```python
from build123d import *

# Parameters (mm, degrees)
SKETCH1_W                                  = 100
SKETCH1_H                                  = 40
BOSS_EXTRUDE1_DEPTH                        = 5
SKETCH2_R                                  = 3
CUT_EXTRUDE1_DEPTH                         = 55.083269132
MIRROR1_AT_THE_SECOND_PLANE_COPY_1_SKETC_R = 3
MIRROR1_AT_THE_SECOND_PLANE_COPY_1_DEPTH   = 55.083269132
FLEX1_START                                = 1.366197724
FLEX1_OUTLINE_W                            = 5
FLEX1_OUTLINE_H                            = 40
FLEX1_DEPTH                                = 48.633802276
FLEX1_START_2                              = -3.633802276
FLEX1_2_OUTLINE_W                          = 46.366197724
FLEX1_2_OUTLINE_H                          = 40
FLEX1_2_OUTLINE_R                          = 3
FLEX1_2_DEPTH                              = 3.907802276
FLEX1_START_3                              = -5
FLEX1_3_OUTLINE_W                          = 46.366197724
FLEX1_3_OUTLINE_H                          = 40
FLEX1_3_OUTLINE_R                          = 3
FLEX1_3_DEPTH                              = 6.366197724
FLEX1_START_4                              = -20
FLEX1_4_DEPTH                              = 40
RIB1_REACH                                 = 79.708
SKETCH3_WALL_W                             = 172.55443254
SKETCH3_WALL_H                             = 3


with BuildPart() as part:
    # Sketch1 → Boss-Extrude1 (new body)
    with BuildSketch(Plane(origin=(0, 0, 0), x_dir=(1, 0, 0), z_dir=(0, 1, 0))):
        Rectangle(SKETCH1_W, SKETCH1_H)
    extrude(amount=BOSS_EXTRUDE1_DEPTH)

    # Sketch2 → Cut-Extrude1 (cut, through all)
    with BuildSketch(Plane(origin=(0, 5, 0), x_dir=(1, 0, 0), z_dir=(0, 1, 0))):
        with Locations(Location((-35, 10, 0), (0, 0, 270))):
            Circle(SKETCH2_R)
    cut_extrude1 = extrude(amount=-CUT_EXTRUDE1_DEPTH, mode=Mode.SUBTRACT)

    # Mirror1: Cut-Extrude1 across plane
    add(cut_extrude1.mirror(Plane.XY), mode=Mode.SUBTRACT)

    # Mirror1 at the second plane: Cut-Extrude1 across plane
    add(cut_extrude1.mirror(Plane(origin=(0, 0, 0), x_dir=(0, 0, 1), z_dir=(1, 0, 0))), mode=Mode.SUBTRACT)

    # Mirror1 at the second plane copy 1 sketc → Mirror1 at the second plane copy 1 (cut, through all)
    with BuildSketch(Plane(origin=(0, 5, 0), x_dir=(-1, 0, 0), z_dir=(0, 1, 0))):
        with Locations(Location((-35, 10, 0), (0, 0, 270))):
            Circle(MIRROR1_AT_THE_SECOND_PLANE_COPY_1_SKETC_R)
    extrude(amount=-MIRROR1_AT_THE_SECOND_PLANE_COPY_1_DEPTH, mode=Mode.SUBTRACT)

    # Flex1: read off the stored shape, not the designer's step
    # Flex1 outline → Flex1 (cut)
    with BuildSketch(Plane.YZ.offset(FLEX1_START)):
        with Locations((2.5, 0)):
            Rectangle(FLEX1_OUTLINE_W, FLEX1_OUTLINE_H)
    extrude(amount=FLEX1_DEPTH, mode=Mode.SUBTRACT)

    # Flex1 2 outline → Flex1 2 (add)
    with BuildSketch(Plane.YZ.offset(FLEX1_START_2)):
        with Locations((28.183098862, 0)):
            Rectangle(FLEX1_2_OUTLINE_W, FLEX1_2_OUTLINE_H)
        with Locations((36.366197724, -10)):
            Circle(FLEX1_2_OUTLINE_R, mode=Mode.SUBTRACT)
        with Locations((36.366197724, 10)):
            Circle(FLEX1_2_OUTLINE_R, mode=Mode.SUBTRACT)
    extrude(amount=FLEX1_2_DEPTH)

    # Flex1 3 outline → Flex1 3 (add)
    with BuildSketch(Plane.YZ.offset(FLEX1_START_3)):
        with Locations((28.183098862, 0)):
            Rectangle(FLEX1_3_OUTLINE_W, FLEX1_3_OUTLINE_H)
        with Locations((36.366197724, -10)):
            Circle(FLEX1_3_OUTLINE_R, mode=Mode.SUBTRACT)
        with Locations((36.366197724, 10)):
            Circle(FLEX1_3_OUTLINE_R, mode=Mode.SUBTRACT)
    extrude(amount=FLEX1_3_DEPTH)

    # Flex1 4 outline → Flex1 4 (cut)
    with BuildSketch(Plane.XY.offset(FLEX1_START_4)):
        with BuildLine():
            Line((1.366197724, 0), (1.366197724, 6.366197724))
            ThreePointArc((1.366197724, 6.366197724), (-0.498418419, 1.864616143), (-5, 0))
            Line((-5, 0), (1.366197724, 0))
        make_face()
        with BuildLine():
            ThreePointArc((-5, 5), (-4.033952325, 5.400150049), (-3.633802276, 6.366197724))
            Line((-3.633802276, 6.366197724), (-3.633802276, 51.366197724))
            Line((-3.633802276, 51.366197724), (-5, 51.366197724))
            Line((-5, 51.366197724), (-5, 5))
        make_face()
    extrude(amount=FLEX1_4_DEPTH, mode=Mode.SUBTRACT)

    # Sketch3 wall → Rib1 (add, up to next)
    with BuildSketch(Plane(origin=(-9.316901138, 10, 10), x_dir=(-0.750787351307, -0.660543982727, 0), z_dir=(0.660543982727, -0.750787351307, 0)), mode=Mode.PRIVATE) as rib1_sk1:
        Rectangle(SKETCH3_WALL_W, SKETCH3_WALL_H)
    rib1_tool1 = extrude(rib1_sk1.sketch, amount=RIB1_REACH, mode=Mode.PRIVATE) - part.part
    rib1 = rib1_tool1.solids().sort_by_distance((-9.316901138, 10, 10))[0]
    add(rib1)

    # Mirror2: Rib1 across plane
    add(rib1.mirror(Plane.XY))


solid = part.part
```
Part model, mm, in its own coordinate system. A direction names the side the tool comes from. Round coordinates to 2 decimals unless told otherwise and drop trailing zeros. Loops run counter-clockwise (first coordinate to the right, second up) from the corner with the lowest first, then second, coordinate; pieces in that order, holes last.
Item 1: Cut at B-B, the plane x = -2. Give the cut face in (y, z).
Item 2: Cut at C-C, the plane z = -18. Give the cut face in (x, y).
Item 3: Mould opens along Z. For faces 1 (the face through (-32.97, 2.54, -12.21)), 2 (the face through (-28, 0, 0)), 3 (the face through (-7, 8, 11.5)) say: +Z half, -Z half, draft (parallel to the pull), parting line (faces both ways), or undercut.
Item 4: Cut at D-D, the plane y = 29. Give the cut face in (x, z).
Item 5: Drill centre lines: line 1 (Z direction, x = -8, y = 10); line 2 (Y direction, x = -14, z = 3.5); line 3 (X direction, y = 27.5, z = -13). Where is each one in solid material? Low to high.
Item 6: Drop flat-ended pins along their axis: P1, Ø20, axis at y = 24, z = -0.5, coming from the -X side; P2, Ø10, axis at y = 15, z = 10.5, coming from the -X side; P3, Ø3, axis at x = -10, y = 8.5, coming from the +Z side. Give the stop position or say it passes through.
Item 7: 3-axis set-ups, long thin cutter, end or side, ignore diameter. For faces 4 (the face through (-7, 8, -11.5)), 5 (the face through (-28, 5, 0)), 6 (the face through (1.366, 29, 0)): which of +Z, -Z, +X, -X, +Y, -Y reach the whole face in a straight line?
Item 8: Cut at A-A, the plane z = 10. Give the cut face in (x, y), then the cut area to 3 significant figures.
A:
1. outline: (0.75, -20) - (51.37, -20) - (51.37, 20) - (0.75, 20) - close; hole circle Ø6 at (36.37, -10); hole circle Ø6 at (36.37, 10)
2. outline: (-50, 0) - (-5, 0) arc R6.37 ccw to (1.37, 6.37) - (1.37, 51.37) - (-3.63, 51.37) - (-3.63, 6.37) arc R1.37 cw to (-5, 5) - (-50, 5) - close
3. face 1: undercut
3. face 2: draft
3. face 3: +Z half
4. outline: (-3.63, -20) - (1.37, -20) - (1.37, 20) - (-3.63, 20) - close
5. line 1: z = -11.5 to -8.5, 8.5 to 11.5
5. line 2: y = 0 to 5
5. line 3: x = -3.63 to 1.37
6. P1: stops at x = -3.63
6. P2: stops at x = -9.32
6. P3: stops at z = 11.5
7. face 4: -Z, -X, +Y
7. face 5: -X, +Y
7. face 6: +Z, -Z, +X, +Y, -Y
8. outline: (-50, 0) - (-38, 0) - (-38, 5) - (-50, 5) - close; (-32, 0) - (-5, 0) arc R6.37 ccw to (1.37, 6.37) - (1.37, 33.37) - (-3.63, 33.37) - (-3.63, 15) - (-15, 5) - (-32, 5) - close; (-3.63, 39.37) - (1.37, 39.37) - (1.37, 51.37) - (-3.63, 51.37) - close
8. area: 477 mm2
